from build123d import *

# Parameters (mm, degrees)
F0_W     = 89.250375
F0_H     = 77.722203
F1_DEPTH = 50.8
F2_R     = 21.558344
F3_DEPTH = 38.1
F4_R     = 16.858314
F5_DEPTH = 127


with BuildPart() as f1:
    # F0 (on Front) → F1 (new body)
    with BuildSketch(Plane.XZ):
        with Locations((1.109326, -1.622727)):
            Rectangle(F0_W, F0_H)
    extrude(amount=F1_DEPTH)

    # F2 (on face) → F3 (join)
    with BuildSketch(Plane.XZ.offset(50.8)):
        Circle(F2_R)
    extrude(amount=F3_DEPTH)

    # F4 (on face) → F5 (cut)
    with BuildSketch(Plane.XZ.offset(88.9)):
        Circle(F4_R)
    extrude(amount=-F5_DEPTH, mode=Mode.SUBTRACT)


solid = f1.part
Verification items for the finished model (mm, model axes). A direction names the side the tool comes from. Give positions to 0.01 mm unless a question says otherwise; leave off trailing zeros. Loops run counter-clockwise (first coordinate to the right, second up) from the corner with the lowest first, then second, coordinate; pieces in that order, holes last.
1. Material ranges on probe 1 along Z at (x, y) = (0, -63); probe 2 along Z at (x, y) = (0, -50); probe 3 along Y at (x, z) = (22, 28.5), recorded low to high.
Derived:
probe 1: z = -21.56 to -16.86, 16.86 to 21.56
probe 2: z = -40.48 to -16.86, 16.86 to 37.24
probe 3: y = -50.8 to 0
2. Cross-section at D-D on z = -24.5. Record the cut outline in (x, y).
Derived:
outline: (-43.52, -50.8) - (45.73, -50.8) - (45.73, 0) - (-43.52, 0) - close
3. Release check for a two-part mould opening along Z. For faces 3 (the cylindrical face through (-4.673, -69.583, -21.046)), 4 (the cylindrical face through (-12.43, -45.07, 11.39)), 5 (the flat face through (-13, -88.9, -11)) record: +Z half, -Z half, draft (parallel to the pull), parting line (faces both ways), or undercut.
Derived:
face 3: parting line
face 4: undercut
face 5: draft
4. Go/stop test with flat-tipped pins: P1, Ø1.5, axis at x = 11, z = -28, coming from the +Y side; P2, Ø2, axis at y = -61, z = -6, coming from the +X side. Record where each tip stops, or that it passes through.
Derived:
P1: stops at y = 0
P2: stops at x = 20.97
5. Cross-section at B-B on z = 0. Record the cut outline in (x, y), and give its area (3 significant figures).
Derived:
outline: (-43.52, -50.8) - (-21.56, -50.8) - (-21.56, -88.9) - (-16.86, -88.9) - (-16.86, 0) - (-43.52, 0) - close; (16.86, -88.9) - (21.56, -88.9) - (21.56, -50.8) - (45.73, -50.8) - (45.73, 0) - (16.86, 0) - close
area: 3,180 mm2
6. Tool access check on faces 1 (the flat face through (0, -25, 37.238)), 2 (the flat face through (20, -50.8, -10)). Record the directions out of +Z, -Z, +X, -X, +Y, -Y that give a thin tool (end or side, any length) a straight path to the whole face; none if there is none.
Derived:
face 1: +Z, +X, -X, +Y, -Y
face 2: -Y
7. Cross-section at C-C on y = -12.5. Record the cut outline in (x, z), and give its area (3 significant figures).
Derived:
outline: (-43.52, -40.48) - (45.73, -40.48) - (45.73, 37.24) - (-43.52, 37.24) - close; hole circle Ø33.72 at (0, 0)
area: 6,040 mm2
8. Cross-section at A-A on x = 0. Record the cut outline in (y, z).
Derived:
outline: (-88.9, -21.56) - (-50.8, -21.56) - (-50.8, -40.48) - (0, -40.48) - (0, -16.86) - (-88.9, -16.86) - close; (-88.9, 16.86) - (0, 16.86) - (0, 37.24) - (-50.8, 37.24) - (-50.8, 21.56) - (-88.9, 21.56) - close
